For this review, use the dimensioned drawing (mm, ordinates from the lowest corner) and the shaded views. Coordinates: 2 decimals unless noted, no trailing zeros. Write each loop counter-clockwise with the first axis right and the second up, starting at its lowest first coordinate (ties: lowest second). Pieces come first, ordered by that corner, then holes. Notation, with made-up numbers: M 63,35.5 L 97,35.5 A14 ccw 97,39.5 Z; hole C -28,-18 d7. An arc over 180 degrees is marked long. Return JSON: item names as keys, results as strings. Group by question number.
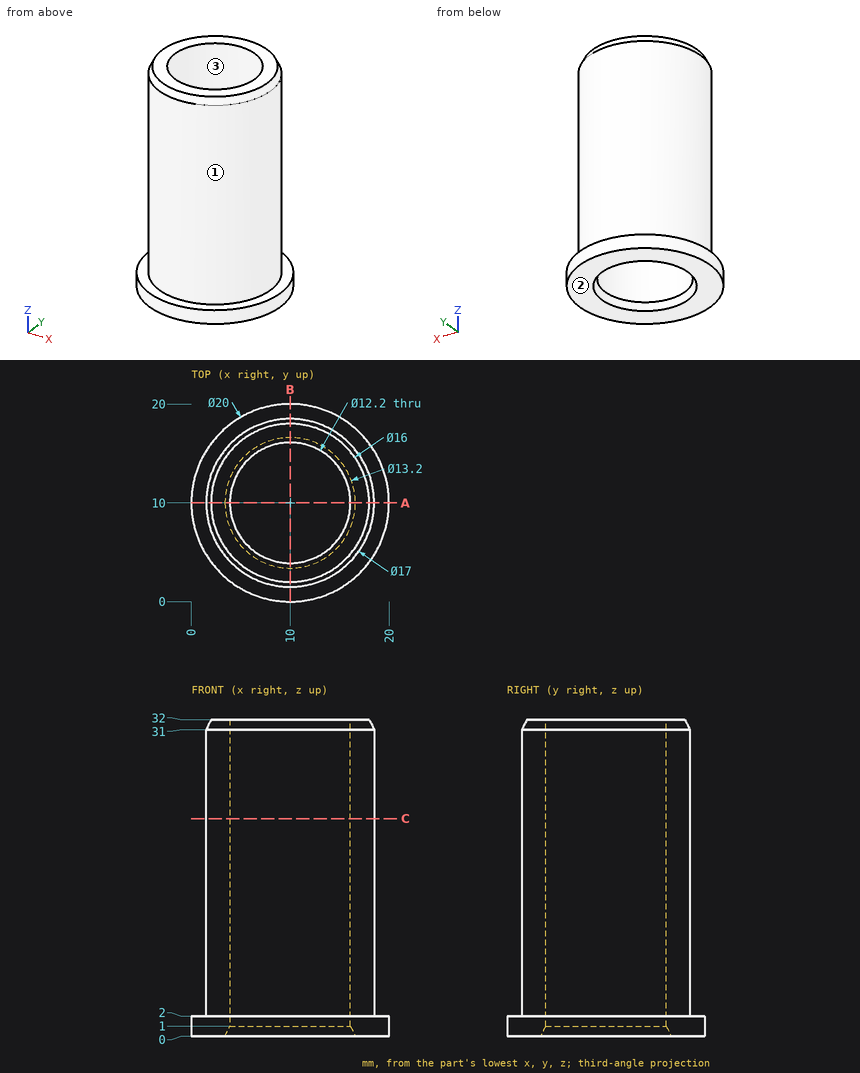
Item 1: For pin 1 (1 mm diameter, centred on y = 7.5, z = 13, fed in from +X); pin 2 (2 mm diameter, centred on x = 8.5, y = 13, fed in from -Z); pin 3 (6 mm diameter, centred on x = 5, z = 27.5, fed in from -Y); pin 4 (5 mm diameter, centred on x = 17.5, z = 8.5, fed in from -Y), all flat-tipped, find the tip position at first contact; note any pin that passes through.
Item 2: Add section A-A (y = 10). Write out the cut boundary in (x, z).
Item 3: Add section C-C (z = 22). Write out the cut boundary in (x, y), plus the area to 3 significant figures.
Item 4: For line 1 (Y direction, x = 10, z = 9); line 2 (Z direction, x = 13.75, y = 18.75), list the stretches that pass through material, from the lowest coordinate up.
Item 5: The part is to be moulded in two halves that separate along X. For the marked faces 1, 2 and 3, say which applies: pulls with the +X half, pulls with the -X half, needs draft (parallel to the pull), parting line crosses it, or undercut.
Geometry check:
{
 "1": {"pin 1": "x = 18.26", "pin 2": "through", "pin 3": "y = 1.74", "pin 4": "y = 3.13"},
 "2": {"outline": "M 0,0 L 3.4,0 L 3.9,1 L 3.9,32 L 2,32 L 1.5,31 L 1.5,2 L 0,2 Z; M 16.1,1 L 16.6,0 L 20,0 L 20,2 L 18.5,2 L 18.5,31 L 18,32 L 16.1,32 Z"},
 "3": {"outline": "C 10,10 d17; hole C 10,10 d12.2", "area": "110 mm^2"},
 "4": {"line 1": "1.5 to 3.9, 16.1 to 18.5", "line 2": "0 to 2"},
 "5": {"face 1": "parting line crosses it", "face 2": "needs draft", "face 3": "undercut"}
}
